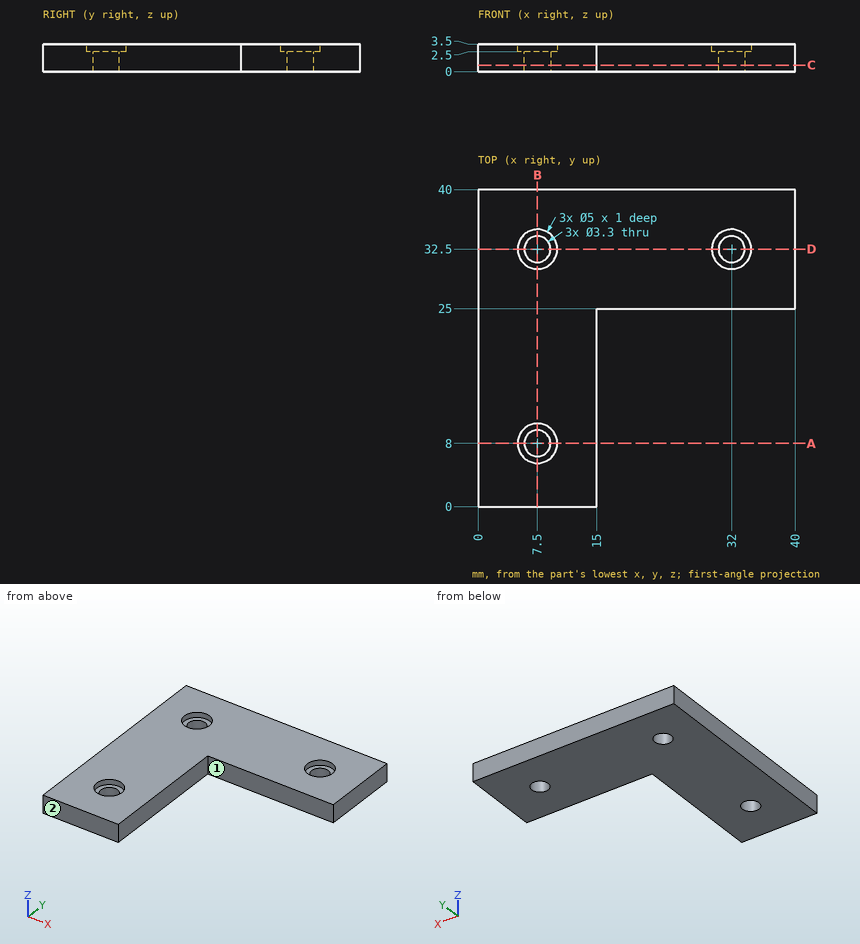
Source: three-view drawing plus pictorial views. Frame: mm from the lowest corner of the part. A direction names the side the tool comes from. Give positions to 0.01 mm unless a question says otherwise; leave off trailing zeros. Order: outer loops, then holes, each group sorted by start corner. A loop starts at its lowest first (then second) coordinate and runs counter-clockwise, first axis right, second up. Notation, with made-up numbers: (67.25, -34.5) -> (118.25, -34.5) arc R23 ccw to (118.25, -0.5) -> close; hole circle Ø10 at (62, -33). An arc over 180 degrees is marked (long way). Put each result on its own line as item: value.
Q1. Section C-C, the plane z = 0.85. Return loops of the section in (x, y).
Here are the results:
outline: (0, 0) -> (15, 0) -> (15, 25) -> (40, 25) -> (40, 40) -> (0, 40) -> close; hole circle Ø3.3 at (7.5, 8); hole circle Ø3.3 at (7.5, 32.5); hole circle Ø3.3 at (32, 32.5)
Q2. Reachability of the marked faces 1 and 2 from +Z, -Z, +X, -X, +Y, -Y: full face, straight path, thin tool, end or side. Return the list, or none.
Here are the results:
face 1: +Z, -Z, +X, -Y
face 2: +Z, -Z, +X, -X, -Y
Q3. Section D-D, the plane y = 32.5. Return loops of the section in (x, z), then the cut area to 4 significant figures.
Here are the results:
outline: (0, 0) -> (5.85, 0) -> (5.85, 2.5) -> (5, 2.5) -> (5, 3.5) -> (0, 3.5) -> close; (9.15, 0) -> (30.35, 0) -> (30.35, 2.5) -> (29.5, 2.5) -> (29.5, 3.5) -> (10, 3.5) -> (10, 2.5) -> (9.15, 2.5) -> close; (33.65, 0) -> (40, 0) -> (40, 3.5) -> (34.5, 3.5) -> (34.5, 2.5) -> (33.65, 2.5) -> close
area: 113.5 mm^2
Q4. Section A-A, the plane y = 8. Return loops of the section in (x, z).
Here are the results:
outline: (0, 0) -> (5.85, 0) -> (5.85, 2.5) -> (5, 2.5) -> (5, 3.5) -> (0, 3.5) -> close; (9.15, 0) -> (15, 0) -> (15, 3.5) -> (10, 3.5) -> (10, 2.5) -> (9.15, 2.5) -> close
Q5. Section B-B, the plane x = 7.5. Return loops of the section in (y, z).
Here are the results:
outline: (0, 0) -> (6.35, 0) -> (6.35, 2.5) -> (5.5, 2.5) -> (5.5, 3.5) -> (0, 3.5) -> close; (9.65, 0) -> (30.85, 0) -> (30.85, 2.5) -> (30, 2.5) -> (30, 3.5) -> (10.5, 3.5) -> (10.5, 2.5) -> (9.65, 2.5) -> close; (34.15, 0) -> (40, 0) -> (40, 3.5) -> (35, 3.5) -> (35, 2.5) -> (34.15, 2.5) -> close
Q6. Material intervals for L1, parallel to Y at x = 7.5, z = 1.75; L2, parallel to Y at x = 7.5, z = 3.3; L3, parallel to Y at x = 32, z = 2.95, sorted ascending.
Here are the results:
L1: y = 0 to 6.35, 9.65 to 30.85, 34.15 to 40
L2: y = 0 to 5.5, 10.5 to 30, 35 to 40
L3: y = 25 to 30, 35 to 40
Q7. Pin query (flat end, axial travel): pin 1 (1.5 mm diameter, centred on x = 32.5, y = 29.5, fed in from -Z); pin 2 (4.5 mm diameter, centred on x = 32, y = 32.5, fed in from +Z); pin 3 (1 mm diameter, centred on x = 24, z = 2, fed in from -Y); pin 4 (3 mm diameter, centred on x = 7.5, y = 8, fed in from +Z). Return the tip coordinate at first contact, or that it passes through.
Here are the results:
pin 1: stops at z = 0
pin 2: stops at z = 2.5
pin 3: stops at y = 25
pin 4: passes through
